Solid Edge part; units mm, degrees
sketch "Sketch1" plane through (0, 0, 0) normal (0, -1, 0) x (1, 0, 0)
  line L0 (-25, -2.5) -> (25, -2.5)
  line L1 (25, -2.5) -> (25, 2.5)
  line L2 (25, 2.5) -> (-25, 2.5)
  line L3 (-25, 2.5) -> (-25, -2.5)
  circle A0 centre (-5.144, 0) radius 1.6
  dimension "D1" = 25
  dimension "D2" = 25
extrude "Protrusion1" add sketch "Sketch1" along normal mid plane 3
hole "Hole_3" at (-22, -1.5, 0) direction (0, 1, 0) diameter 3.2 end up to next
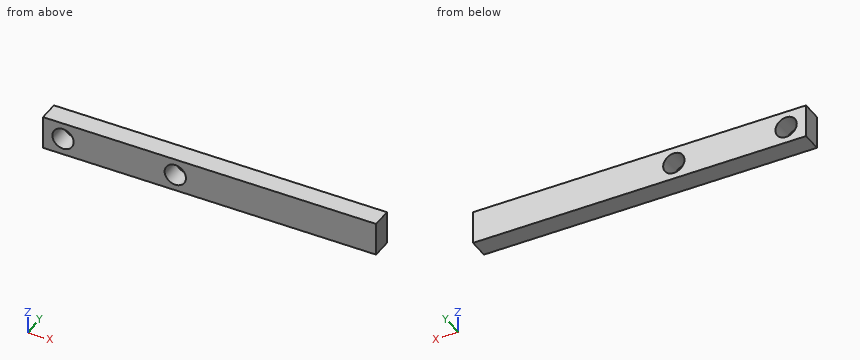
For this review, take the finished solid that the model builds, in its own axes (mm). Coordinates: 2 decimals unless noted, no trailing zeros. Order: outer loops, then holes, each group sorted by start corner. A loop starts at its lowest first (then second) coordinate and runs counter-clockwise, first axis right, second up. Notation, with made-up numbers: (5.25, 53) - (10.25, 53) arc R12 cw to (10.25, 64) - close; hole circle Ø9 at (-31, 17). An arc over 180 degrees is marked (long way). Answer as CSV lines item,"result". Start each with the question number.
1) Add section A-A (z = 0). State the section outline as (x, y) points, then the cut area to 3 significant figures.
2) Add section C-C (y = 1). State the section outline as (x, z) points, then the cut area to 3 significant figures.
3) Add section B-B (x = -22). State the section outline as (y, z) points.
4) To check wall thickness, follow line 1 along X through (y, z) = (1.35, -0.5); line 2 along X through (y, z) = (0.2, 1.4); line 3 along Z through (x, y) = (-5, -0.5). State the ranges of each line that lie inside material, in increasing order. Write a range as [from, to].
Result:
1,outline,"(-25, -1.5) - (-23.6, -1.5) - (-23.6, 1.5) - (-25, 1.5) - close; (-20.4, -1.5) - (-6.74, -1.5) - (-6.74, 1.5) - (-20.4, 1.5) - close; (-3.54, -1.5) - (25, -1.5) - (25, 1.5) - (-3.54, 1.5) - close"
1,area,"131 mm^2"
2,outline,"(-25, -2.5) - (25, -2.5) - (25, 2.5) - (-25, 2.5) - close; hole circle Ø3.2 at (-22, 0); hole circle Ø3.2 at (-5.14, 0)"
2,area,"234 mm^2"
3,outline,"(-1.5, -2.5) - (1.5, -2.5) - (1.5, -1.6) - (-1.5, -1.6) - close; (-1.5, 1.6) - (1.5, 1.6) - (1.5, 2.5) - (-1.5, 2.5) - close"
4,line 1,"[-25, -23.52], [-20.48, -6.66], [-3.62, 25]"
4,line 2,"[-25, -22.77], [-21.23, -5.92], [-4.37, 25]"
4,line 3,"[-2.5, -1.59], [1.59, 2.5]"
